Geometry: final body of the model. Coordinates: model frame, mm. Face numbers are marked on the shaded views. A direction names the side the tool comes from. Give positions to 0.01 mm unless a question says otherwise; leave off trailing zeros. Write each loop counter-clockwise with the first axis right and the second up, starting at its lowest first coordinate (ties: lowest second). Pieces come first, ordered by that corner, then holes. Notation, with made-up numbers: (2.25, 37) -> (38.25, 37) arc R26 cw to (38.25, 52) -> close; hole circle Ø3 at (-11.75, -38). An arc over 180 degrees is marked (long way). Answer in a Markdown table with one row per item. Add a question column.
Item 1: Section query B-B on z = 28. Output: boundary loops of the cut face in (x, y).
Item 2: Draft query along Y for the marked faces 4, 5 and 6. Return one class per face: +Y half, -Y half, draft (parallel to the pull), parting line (faces both ways), or undercut.
Item 3: Access query for the marked faces 1, 2 and 3. Directions: +Z, -Z, +X, -X, +Y, -Y. A direction counts if a zero-diameter tool reaches every point of the face in a straight line with its end or side. Return the directions, or none.
Item 4: First-contact query: P1, Ø3, axis at x = 23.5, y = 9.5, coming from the +Z side; P2, Ø14.5, axis at x = 11.1, z = 19.5, coming from the +Y side; P3, Ø16.5, axis at x = 11.1, z = 19.5, coming from the -Y side. Flat tips, straight axial feed; report the tip coordinate or a pass-through.
Item 5: Section query A-A on x = 11.1. Output: boundary loops of the cut face in (y, z), plus the area to 3 significant figures.
Item 6: Material intervals for probe 1 along Z at (x, y) = (11.1, 31.65); probe 2 along Y at (x, z) = (46, 6); probe 3 along Y at (x, z) = (9.5, 11.5), sorted ascending. Write a range as from..to.
Item 7: Section query C-C on y = 22.5. Output: boundary loops of the cut face in (x, z).
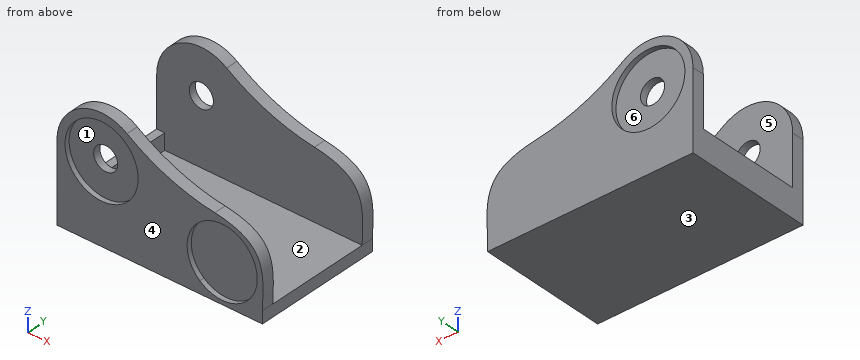
```python
from build123d import *

# Parameters (mm, degrees)
F0_R            = 9.1
F0_W            = 2
F0_H            = 4
F0_R_2          = 3
F1_DEPTH        = 3
F1_COPIES_COUNT = 2
F1_COPIES_PITCH = 29
F2_DEPTH        = 32
F3_R            = 9.1
F4_DEPTH        = 3
F5_DEPTH        = 1.2
F3_R_2          = 3
F6_DEPTH        = 1.2


# Not quite as in the source:
# - a pattern or mirror of a feature is missing from the dataset's text; its kind, count and spacing are read off the source's solid


with BuildPart() as f1:
    # F0 (on Front) → F1 (new body)
    with BuildSketch(Plane.XZ):
        with BuildLine():
            Line((46.6587768439, 3), (51.1, 3))
            add(Edge.make_bspline(
                [(39.2721801194, 20.2002895195), (43.2600263156, 19.672514392), (52.7768717224, 16.5297183629), (51.1, 6.6124380804), (51.1, 3)],
                knots=[0.3415991708, 0.3415991708, 0.3415991708, 0.3415991708, 0.5830024084, 1, 1, 1, 1], degree=3))
            ThreePointArc((39.2721801194, 20.2002895195), (27.8400722418, 23.1174494268), (17.4097910893, 28.6321704107))
            ThreePointArc((17.4097910893, 28.6321704107), (5.9438716604, 29.329768082), (0, 19.5))
            Line((0, 19.5), (0, 7))
            Line((0, 7), (2, 7))
            Line((2, 7), (2, 3))
            Line((2, 3), (35.5412231561, 3))
            ThreePointArc((35.5412231561, 3), (37.3834628323, 17.6188568825), (49.825, 9.725))
            ThreePointArc((49.825, 9.725), (48.9938568825, 6.0084628323), (46.6587768439, 3))
        make_face()
        with Locations((11.1, 19.5)):
            Circle(F0_R, mode=Mode.SUBTRACT)
        with Locations((1, 5)):
            Rectangle(F0_W, F0_H)
        with BuildLine():
            Line((0, 3), (0, 0))
            Line((0, 0), (51.1, 0))
            Line((51.1, 0), (51.1, 3))
            Line((51.1, 3), (46.6587768439, 3))
            ThreePointArc((46.6587768439, 3), (41.1, 1), (35.5412231561, 3))
            Line((35.5412231561, 3), (2, 3))
            Line((2, 3), (0, 3))
        make_face()
        with BuildLine():
            Line((35.5412231561, 3), (46.6587768439, 3))
            ThreePointArc((46.6587768439, 3), (48.9938568825, 6.0084628323), (49.825, 9.725))
            ThreePointArc((49.825, 9.725), (37.3834628323, 17.6188568825), (35.5412231561, 3))
        make_face()
        with BuildLine():
            ThreePointArc((35.5412231561, 3), (41.1, 1), (46.6587768439, 3))
            Line((46.6587768439, 3), (35.5412231561, 3))
        make_face()
        with Locations((11.1, 19.5)):
            Circle(F0_R)
        with Locations((11.1, 19.5)):
            Circle(F0_R_2, mode=Mode.SUBTRACT)
    extrude(amount=-F1_DEPTH)


with BuildPart() as f1_copies_1:
    # F1_copies: instance of F1
    add(f1.part.moved(Location(Vector(0, 1, 0) * (1 * F1_COPIES_PITCH))))


with BuildPart() as f1_1:
    add(f1.part)

    add(f1_copies_1.part)  # F2 merges F1_copies_1
    # F0 (on Front) → F2 (join)
    with BuildSketch(Plane.XZ):
        with BuildLine():
            ThreePointArc((35.5412231561, 3), (41.1, 1), (46.6587768439, 3))
            Line((46.6587768439, 3), (35.5412231561, 3))
        make_face()
        with BuildLine():
            Line((0, 3), (0, 0))
            Line((0, 0), (51.1, 0))
            Line((51.1, 0), (51.1, 3))
            Line((51.1, 3), (46.6587768439, 3))
            ThreePointArc((46.6587768439, 3), (41.1, 1), (35.5412231561, 3))
            Line((35.5412231561, 3), (2, 3))
            Line((2, 3), (0, 3))
        make_face()
        with Locations((1, 5)):
            Rectangle(F0_W, F0_H)
    extrude(amount=-F2_DEPTH)

    # F3 (on face) → F4 (join)
    with BuildSketch(Plane(origin=(0, 32, 0), x_dir=(-1, 0, 0), z_dir=(0, 1, 0))):
        with BuildLine():
            Line((-35.5412231561, 3), (-2, 3))
            Line((-2, 3), (-2, 7))
            Line((-2, 7), (0, 7))
            Line((0, 7), (0, 19.5))
            ThreePointArc((0, 19.5), (-5.9438716604, 29.329768082), (-17.4097910893, 28.6321704107))
            ThreePointArc((-17.4097910893, 28.6321704107), (-24.6422981145, 24.4802718869), (-32.4642883797, 21.5882332434))
            ThreePointArc((-32.4642883797, 21.5882332434), (-35.8440967329, 20.7758663792), (-39.2721801194, 20.2002895195))
            add(Edge.make_bspline(
                [(-39.2721801194, 20.2002895195), (-43.2600263156, 19.672514392), (-50.5817963384, 17.2546092175), (-51.2780387876, 10.8269071453), (-51.2543959351, 7.7483589961)],
                knots=[0.3415991708, 0.3415991708, 0.3415991708, 0.3415991708, 0.5830024084, 0.8481388116, 0.8481388116, 0.8481388116, 0.8481388116], degree=3))
            add(Edge.make_bspline(
                [(-51.1, 3), (-50.9854700291, 4.1577635436), (-50.9621826453, 5.7020696678), (-51.1914335387, 7.3646437275), (-51.2543959351, 7.7483589961)],
                knots=[0, 0, 0, 0, 3.6124380804, 4.6797314617, 4.6797314617, 4.6797314617, 4.6797314617], degree=3))
            Line((-51.1, 3), (-46.6587768439, 3))
            ThreePointArc((-46.6587768439, 3), (-41.1, 18.45), (-35.5412231561, 3))
        make_face()
        with Locations((-11.1, 19.5)):
            Circle(F3_R, mode=Mode.SUBTRACT)
        with BuildLine():
            Line((-46.6587768439, 3), (-35.5412231561, 3))
            ThreePointArc((-35.5412231561, 3), (-41.1, 18.45), (-46.6587768439, 3))
        make_face()
    extrude(amount=-F4_DEPTH)

    # F0 (on Front) → F5 (cut)
    with BuildSketch(Plane.XZ):
        with Locations((11.1, 19.5)):
            Circle(F0_R)
        with Locations((11.1, 19.5)):
            Circle(F0_R_2, mode=Mode.SUBTRACT)
        with BuildLine():
            Line((35.5412231561, 3), (46.6587768439, 3))
            ThreePointArc((46.6587768439, 3), (48.9938568825, 6.0084628323), (49.825, 9.725))
            ThreePointArc((49.825, 9.725), (37.3834628323, 17.6188568825), (35.5412231561, 3))
        make_face()
        with BuildLine():
            ThreePointArc((35.5412231561, 3), (41.1, 1), (46.6587768439, 3))
            Line((46.6587768439, 3), (35.5412231561, 3))
        make_face()
    extrude(amount=-F5_DEPTH, mode=Mode.SUBTRACT)

    # F3 (on face) → F6 (cut)
    with BuildSketch(Plane(origin=(0, 32, 0), x_dir=(-1, 0, 0), z_dir=(0, 1, 0))):
        with Locations((-11.1, 19.5)):
            Circle(F3_R)
        with Locations((-11.1, 19.5)):
            Circle(F3_R_2, mode=Mode.SUBTRACT)
    extrude(amount=-F6_DEPTH, mode=Mode.SUBTRACT)


solid = f1_1.part
```
Findings below:
| question | item | result |
|---|---|---|
| 1 | outline | (3.96, 0) -> (7.85, 0) -> (7.85, 1.2) -> (14.35, 1.2) -> (14.35, 0) -> (18.35, 0) -> (18.35, 3) -> (3.96, 3) -> close; (3.96, 29) -> (18.35, 29) -> (18.35, 32) -> (14.35, 32) -> (14.35, 30.8) -> (7.85, 30.8) -> (7.85, 32) -> (3.96, 32) -> close |
| 2 | face 4 | -Y half |
| 2 | face 5 | undercut |
| 2 | face 6 | +Y half |
| 3 | face 1 | -Y |
| 3 | face 2 | +Z, +X |
| 3 | face 3 | -Z, +X, -X, +Y, -Y |
| 4 | P1 | stops at z = 3 |
| 4 | P2 | stops at y = 30.8 |
| 4 | P3 | stops at y = 1.2 |
| 5 | outline | (0, 0) -> (32, 0) -> (32, 10.4) -> (30.8, 10.4) -> (30.8, 16.5) -> (29, 16.5) -> (29, 3) -> (3, 3) -> (3, 16.5) -> (1.2, 16.5) -> (1.2, 10.4) -> (0, 10.4) -> close; (0, 28.6) -> (1.2, 28.6) -> (1.2, 22.5) -> (3, 22.5) -> (3, 30.6) -> (0, 30.6) -> close; (29, 22.5) -> (30.8, 22.5) -> (30.8, 28.6) -> (32, 28.6) -> (32, 30.6) -> (29, 30.6) -> close |
| 5 | area | 196 mm^2 |
| 6 | probe 1 | z = 0..10.4, 28.6..30.6 |
| 6 | probe 2 | y = 1.2..3, 29..32 |
| 6 | probe 3 | y = 1.2..3, 29..30.8 |
| 7 | outline | (0, 0) -> (51.1, 0) -> (51.1, 3) -> (2, 3) -> (2, 7) -> (0, 7) -> close |
